Job drawing, mm, ordinate dimensions from the low corner. One solid piece. A direction names the side the tool comes from. Coordinates: 2 decimals unless noted, no trailing zeros. Loops run counter-clockwise (first coordinate to the right, second up) from the corner with the lowest first, then second, coordinate; pieces in that order, holes last. Notation, with made-up numbers: (51.25, -34.5) -> (64.25, -34.5) arc R34 ccw to (64.25, 1.5) -> close; hole circle Ø6 at (28.25, -0.5). An arc over 180 degrees is marked (long way). Answer as CSV lines item,"result". Start each with the question number.
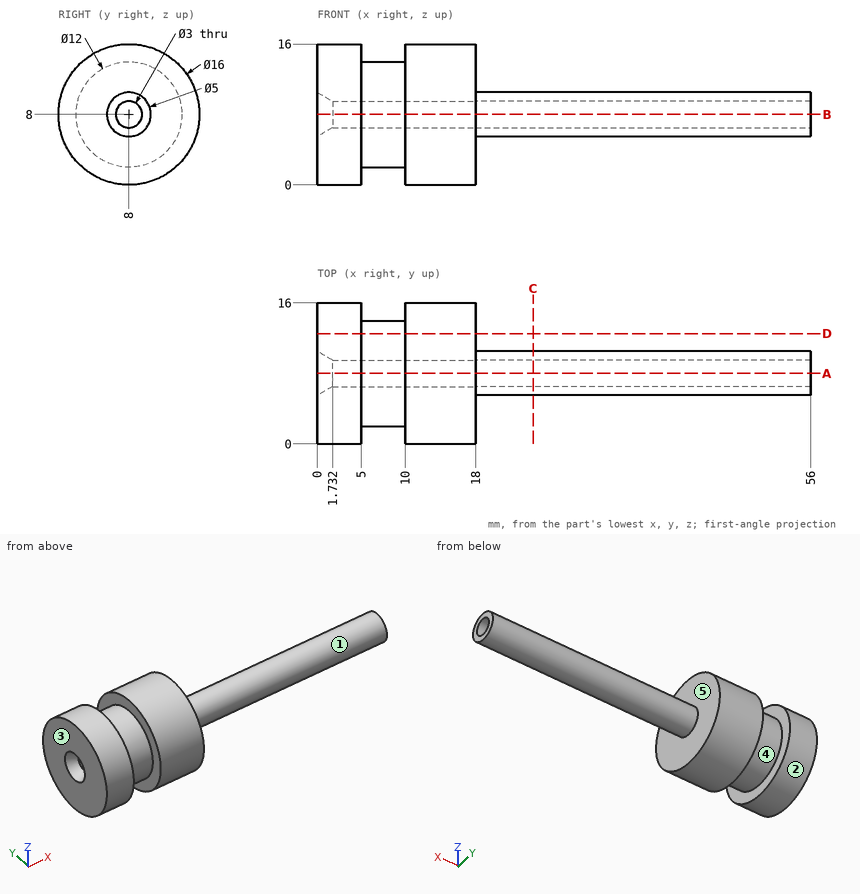
Item 1: Saw through at D-D (y = 12.5). Write the cut outline in (x, z).
Item 2: Wall check: probe 1 along Y at (x, z) = (39.5, 8); probe 2 along Y at (x, z) = (13.75, 8); probe 3 along X at (y, z) = (14.25, 5). Give the ranges that are in metal, low to high.
Item 3: Flat gauge pins, fed straight in: pin 1 Ø1.5 at (x, z) = (37, 6) entering from -Y (3 decimals); pin 2 Ø8 at (x, z) = (47, 11.5) entering from +Y; pin 3 Ø2 at (x, y) = (19.5, 8.5) entering from -Z; pin 4 Ø4 at (y, z) = (10.5, 10) entering from -X. Where does each tip first touch, or does it go through?
Item 4: Saw through at C-C (x = 24.5). Write the cut outline in (y, z), plus the area to 3 significant figures.
Item 5: Two-plate mould, pull along X, no slides. Class the marked faces 3, 4 and 5: pulls with the +X half, pulls with the -X half, needs draft (parallel to the pull), parting line crosses it, or undercut.
Item 6: Saw through at A-A (y = 8). Write the cut outline in (x, z).
Item 7: Which spindle directions (+Z, -Z, +X, -X, +Y, -Y) get a long thin tool onto all of the face, cutting with end or side? Do the marked faces 1 and 2. Say none if no direction does.
Geometry check:
1,outline,"(0, 1.39) -> (5, 1.39) -> (5, 4.03) -> (10, 4.03) -> (10, 1.39) -> (18, 1.39) -> (18, 14.61) -> (10, 14.61) -> (10, 11.97) -> (5, 11.97) -> (5, 14.61) -> (0, 14.61) -> close"
2,probe 1,"5.5 to 6.5, 9.5 to 10.5"
2,probe 2,"0 to 6.5, 9.5 to 16"
2,probe 3,"0 to 5, 10 to 18"
3,pin 1,"y = 5.835"
3,pin 2,"y = 10.5"
3,pin 3,"z = 5.5"
3,pin 4,"x = 0"
4,outline,"circle Ø5 at (8, 8); hole circle Ø3 at (8, 8)"
4,area,"12.6 mm2"
5,face 3,"pulls with the -X half"
5,face 4,"undercut"
5,face 5,"pulls with the +X half"
6,outline,"(0, 0) -> (5, 0) -> (5, 2) -> (10, 2) -> (10, 0) -> (18, 0) -> (18, 5.5) -> (56, 5.5) -> (56, 6.5) -> (1.73, 6.5) -> (0, 5.5) -> close; (0, 10.5) -> (1.73, 9.5) -> (56, 9.5) -> (56, 10.5) -> (18, 10.5) -> (18, 16) -> (10, 16) -> (10, 14) -> (5, 14) -> (5, 16) -> (0, 16) -> close"
7,face 1,"+X"
7,face 2,"+X, -X"
